from build123d import *

# Parameters (mm, degrees)
SKETCH_R     = 2.8
PAD_DEPTH    = 3
SKETCH001_R  = 1.45
PAD001_DEPTH = 25
POCKET_DEPTH = 2
CHAMFER_SIZE = 0.25


with BuildPart() as part:
    # Sketch → Pad (new body)
    with BuildSketch(Plane.XY):
        Circle(SKETCH_R)
    extrude(amount=PAD_DEPTH)

    # Sketch001 (on Face3 of Pad) → Pad001 (join)
    with BuildSketch(Plane.XY.offset(3)):
        Circle(SKETCH001_R)
    extrude(amount=PAD001_DEPTH)

    # Sketch002 (on Face2 of Pad001) → Pocket (cut)
    with BuildSketch(Plane(origin=(0, 0, 0), x_dir=(1, 0, 0), z_dir=(0, 0, -1))):
        Polygon((1.259542, 0.814588), (-0.075682, 1.49809), (-1.335225, 0.683502), (-1.259542, -0.814588), (0.075682, -1.49809), (1.335225, -0.683502), align=None)
    extrude(amount=-POCKET_DEPTH, mode=Mode.SUBTRACT)

    # Chamfer
    chamfer_edges = [part.edges().sort_by_distance(p)[0] for p in [
        (-2.8, 0, 3),
        (-2.8, 0, 0),
        (1.297384, -0.065543, 0),
        (0.705454, 1.090796, 0),
        (-0.59193, 1.156339, 0),
        (-1.297384, 0.065543, 0),
        (-0.705454, -1.090796, 0),
        (0.59193, -1.156339, 0),
        (-1.45, 0, 28),
    ]]
    chamfer(chamfer_edges, length=CHAMFER_SIZE)


solid = part.part
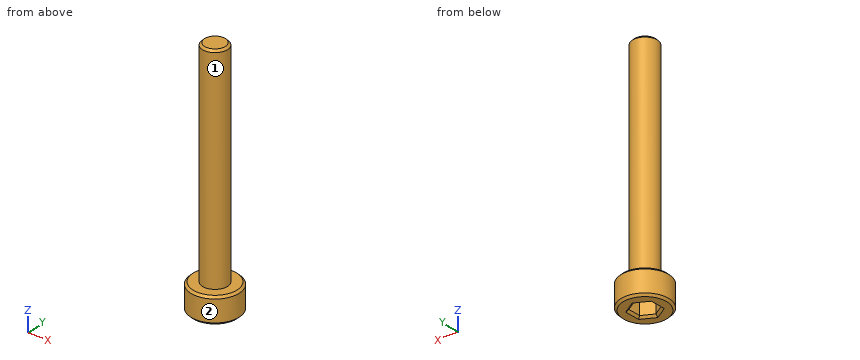
Read the model definition and answer for the solid it produces. Units are mm, in the model's axes. Face numbers are marked on the shaded views. A direction names the side the tool comes from. Round coordinates to 2 decimals unless told otherwise and drop trailing zeros. Loops run counter-clockwise (first coordinate to the right, second up) from the corner with the lowest first, then second, coordinate; pieces in that order, holes last.
Q1. Consider probe 1 along Y at (x, z) = (1.2, 24.25); probe 2 along Z at (x, y) = (-2.5, 0.4); probe 3 along Z at (x, y) = (0.55, 0.75). Determine where each line is inside the solid, lowest interval first.
Q2. Each of these flat-tipped pins is pushed along its axis until it touches: pin 1 (1 mm diameter, centred on x = 2, y = -2, fed in from +Z); pin 2 (0.8 mm diameter, centred on x = 0, y = 0, fed in from -Z); pin 3 (1.5 mm diameter, centred on x = -1.5, z = 14.5, fed in from -Y). Where does it stop, or does it pass through?
Q3. Section B-B on y = 0 is taken. Write down the section's boundary in (x, z), and give its area (3 significant figures).
Q4. Section A-A on z = 11 is taken. Write down the section's boundary in (x, y), and give its area (3 significant figures).
Q5. Which of the six approach directions +Z, -Z, +X, -X, +Y, -Y give full straight-line access (tool end or side, diameter ignored) to the marked faces 1 and 2?
Output:
1. probe 1: y = -0.81 to 0.81
1. probe 2: z = 0 to 3
1. probe 3: z = 2 to 28
2. pin 1: stops at z = 3
2. pin 2: stops at z = 2
2. pin 3: stops at y = -1.24
3. outline: (-2.8, 0.25) - (-2.55, 0) - (-1.55, 0) - (-1.3, 0.25) - (-1.3, 2) - (1.3, 2) - (1.3, 0.25) - (1.55, 0) - (2.55, 0) - (2.8, 0.25) - (2.8, 2.75) - (2.55, 3) - (1.45, 3) - (1.45, 27.75) - (1.2, 28) - (-1.2, 28) - (-1.45, 27.75) - (-1.45, 3) - (-2.55, 3) - (-2.8, 2.75) - close
3. area: 83.8 mm2
4. outline: circle Ø2.9 at (0, 0)
4. area: 6.61 mm2
5. face 1: +Z
5. face 2: +Z, -Z
